Here's how the part is built. I have some questions about the finished solid (model axes, mm). A direction names the side the tool comes from. Round coordinates to 2 decimals unless told otherwise and drop trailing zeros. Order: outer loops, then holes, each group sorted by start corner. A loop starts at its lowest first (then second) coordinate and runs counter-clockwise, first axis right, second up. Notation, with made-up numbers: (17, -25) - (24, -25) arc R23 cw to (24, 2) - close; hole circle Ø2 at (28.5, 60.25). An arc over 180 degrees is marked (long way). Answer as a JSON object with one key per item and string values.
```python
from build123d import *

# Parameters (mm, degrees)
F0_W     = 163
F0_H     = 140
F0_W_2   = 123
F0_H_2   = 100
F0_W_3   = 115
F0_H_3   = 92
F1_DEPTH = 3
F2_W     = 163
F2_H     = 140
F2_W_2   = 157
F2_H_2   = 134
F3_DEPTH = 40
F4_R     = 5
F5_R     = 2
F6_SIZE  = 0.25
F7_SIZE  = 1


with BuildPart() as f1:
    # F0 (on Top) → F1 (new body)
    with BuildSketch(Plane.XY):
        Rectangle(F0_W, F0_H)
        Rectangle(F0_W_2, F0_H_2, mode=Mode.SUBTRACT)
        Rectangle(F0_W_2, F0_H_2)
        Rectangle(F0_W_3, F0_H_3, mode=Mode.SUBTRACT)
        Rectangle(F0_W_3, F0_H_3)
    extrude(amount=F1_DEPTH)

    # F2 (on face) → F3 (join)
    with BuildSketch(Plane.XY.offset(3)):
        Rectangle(F2_W, F2_H)
        Rectangle(F2_W_2, F2_H_2, mode=Mode.SUBTRACT)
    extrude(amount=F3_DEPTH)

    # F4
    f4_edges = [f1.edges().sort_by_distance(p)[0] for p in [
        (-81.5, -70, 21.5),
        (81.5, -70, 21.5),
        (81.5, 70, 21.5),
        (-81.5, 70, 21.5),
    ]]
    fillet(f4_edges, radius=F4_R)

    # F5
    f5_edges = [f1.edges().sort_by_distance(p)[0] for p in [
        (78.5, -67, 23),
        (-78.5, -67, 23),
        (78.5, 67, 23),
        (-78.5, 67, 23),
    ]]
    fillet(f5_edges, radius=F5_R)

    # F6
    f6_edges = [f1.edges().sort_by_distance(p)[0] for p in [
        (0, -70, 0),
        (-80.035534, -68.535534, 0),
        (80.035534, -68.535534, 0),
        (-81.5, 0, 0),
        (81.5, 0, 0),
        (-80.035534, 68.535534, 0),
        (80.035534, 68.535534, 0),
        (0, 70, 0),
    ]]
    chamfer(f6_edges, length=F6_SIZE)

    # F7
    f7_edges = [f1.edges().sort_by_distance(p)[0] for p in [
        (0, -67, 3),
        (77.914214, -66.414214, 3),
        (-77.914214, -66.414214, 3),
        (78.5, 0, 3),
        (-78.5, 0, 3),
        (77.914214, 66.414214, 3),
        (-77.914214, 66.414214, 3),
        (0, 67, 3),
    ]]
    chamfer(f7_edges, length=F7_SIZE)


solid = f1.part
```
1. Imagine slicing it at A-A (z = 16). List the corners of the cut face in (x, y) for me, plus the area to 3 significant figures.
Responses:
{"outline": "(-81.5, -65) arc R5 ccw to (-76.5, -70) - (76.5, -70) arc R5 ccw to (81.5, -65) - (81.5, 65) arc R5 ccw to (76.5, 70) - (-76.5, 70) arc R5 ccw to (-81.5, 65) - close; hole (-78.5, -65) arc R2 ccw to (-76.5, -67) - (76.5, -67) arc R2 ccw to (78.5, -65) - (78.5, 65) arc R2 ccw to (76.5, 67) - (-76.5, 67) arc R2 ccw to (-78.5, 65) - close", "area": "1,760 mm2"}
2. Imagine slicing it at B-B (y = -45.5). List the corners of the cut face in (x, z) for me, plus the area to 3 significant figures.
Responses:
{"outline": "(-81.5, 0.25) - (-81.25, 0) - (81.25, 0) - (81.5, 0.25) - (81.5, 43) - (78.5, 43) - (78.5, 4) - (77.5, 3) - (-77.5, 3) - (-78.5, 4) - (-78.5, 43) - (-81.5, 43) - close", "area": "730 mm2"}
3. Thinking about a two-plate mould opening in X: for faces 3 (the face through (-79.91, 68.48, 0.12)), 4 (the face through (-1, 1, 0)), 5 (the face through (78.5, -1, 23)), which applies, pulls with the +X half, pulls with the -X half, needs draft (parallel to the pull), parting line crosses it, or undercut?
Responses:
{"face 3": "pulls with the -X half", "face 4": "needs draft", "face 5": "undercut"}
4. If I drill on L1, parallel to X at y = -50.5, z = 20; L2, parallel to Y at x = 17, z = 6.5; L3, parallel to Z at x = 12.5, y = 2.5, over which ranges is the centre line in solid material (lowest first)? Write a range as [from, to].
Responses:
{"L1": "[-81.5, -78.5], [78.5, 81.5]", "L2": "[-70, -67], [67, 70]", "L3": "[0, 3]"}
5. For faces 1 (the face through (-80.07, -68.5, 21.92)), 2 (the face through (-78.5, -1, 23)), which set-ups out of +Z, -Z, +X, -X, +Y, -Y let a thin tool reach every point of the face, with its end or its side?
Responses:
{"face 1": "+Z, -Z, -X, -Y", "face 2": "+Z"}
6. Imagine slicing it at C-C (x = -63.5). List the corners of the cut face in (y, z) for me.
Responses:
{"outline": "(-70, 0.25) - (-69.75, 0) - (69.75, 0) - (70, 0.25) - (70, 43) - (67, 43) - (67, 4) - (66, 3) - (-66, 3) - (-67, 4) - (-67, 43) - (-70, 43) - close"}
